```python
from build123d import *

# Parameters (mm, degrees)
SKETCH1_W             = 105.41
SKETCH1_H             = 114.3
BOSS_EXTRUDE1_DEPTH   = 3.175
F_8_CLEARANCE_HOLE1_D = 4.4958
MIRROR2_COPY_1_D      = 4.4958
CUT_EXTRUDE4_REACH    = 80.002
SKETCH15_W            = 41.275
SKETCH15_H            = 79.375
CUT_EXTRUDE5_REACH    = 80.002
SKETCH17_R            = 1.5875
CUT_EXTRUDE6_DEPTH    = 6.35


with BuildPart() as part:
    # Sketch1 → Boss-Extrude1 (new, symmetric)
    with BuildSketch(Plane(origin=(0, 0, 0), x_dir=(1, 0, 0), z_dir=(0, 1, 0))):
        Rectangle(SKETCH1_W, SKETCH1_H)
    extrude(amount=BOSS_EXTRUDE1_DEPTH, both=True)

    # #8 Clearance Hole1 (through all)
    with Locations(Plane(origin=(0, 3.175, 0), x_dir=(1, 0, 0), z_dir=(0, 1, 0))):
        with Locations((-46.355, 50.8)):
            f_8_clearance_hole1 = Hole(F_8_CLEARANCE_HOLE1_D / 2)

    # Mirror1: #8 Clearance Hole1 across plane
    add(f_8_clearance_hole1.mirror(Plane.XY), mode=Mode.SUBTRACT)

    # Mirror2: #8 Clearance Hole1 across plane
    add(f_8_clearance_hole1.mirror(Plane(origin=(0, 0, 0), x_dir=(0, 0, 1), z_dir=(1, 0, 0))), mode=Mode.SUBTRACT)

    # Mirror2 copy 1 (through all)
    with Locations(Plane(origin=(0, 3.175, 0), x_dir=(-1, 0, 0), z_dir=(0, 1, 0))):
        with Locations((-46.355, 50.8)):
            Hole(MIRROR2_COPY_1_D / 2)

    # Sketch15 → Cut-Extrude4 (cut, up to next)
    with BuildSketch(Plane.XZ.offset(3.175), mode=Mode.PRIVATE) as cut_extrude4_sk1:
        with Locations((6.6675, 4.7625)):
            Rectangle(SKETCH15_W, SKETCH15_H)
    cut_extrude4_tool1 = extrude(cut_extrude4_sk1.sketch, amount=-CUT_EXTRUDE4_REACH, mode=Mode.PRIVATE) & part.part
    add(cut_extrude4_tool1.solids().sort_by_distance((6.6675, -3.175, 4.7625))[0], mode=Mode.SUBTRACT)

    # Sketch16 → Cut-Extrude5 (cut, up to next)
    with BuildSketch(Plane(origin=(0, 3.175, 0), x_dir=(1, 0, 0), z_dir=(0, 1, 0)), mode=Mode.PRIVATE) as cut_extrude5_sk1:
        Polygon((-52.705, -6.35), (-52.705, 6.35), (-46.355, 6.35), (-46.355, 1.89865), (-42.8545625, 1.89865), (-42.8545625, 3.96875), (-40.0764375, 3.96875), (-40.0764375, 1.89865), (-36.576, 1.89865), (-36.576, -1.89865), (-40.0764375, -1.89865), (-40.0764375, -3.96875), (-42.8545625, -3.96875), (-42.8545625, -1.89865), (-46.355, -1.89865), (-46.355, -6.35), align=None)
    cut_extrude5_tool1 = extrude(cut_extrude5_sk1.sketch, amount=-CUT_EXTRUDE5_REACH, mode=Mode.PRIVATE) & part.part
    add(cut_extrude5_tool1.solids().sort_by_distance((-46.496113, 3.175, 0))[0], mode=Mode.SUBTRACT)

    # Sketch17 → Cut-Extrude6 (cut)
    with BuildSketch(Plane(origin=(0, 3.175, 0), x_dir=(1, 0, 0), z_dir=(0, 1, 0))):
        with Locations(Location((-17.145, 28.575, 0), (0, 0, 270))):
            Circle(SKETCH17_R)
        with Locations(Location((-17.145, -38.1, 0), (0, 0, 270))):
            Circle(SKETCH17_R)
        with Locations(Location((30.48, -38.1, 0), (0, 0, 90))):
            Circle(SKETCH17_R)
        with Locations(Location((30.48, 28.575, 0), (0, 0, 90))):
            Circle(SKETCH17_R)
        Polygon((-20.32, 8.73125), (-13.97, 8.73125), (-13.97, 21.43125), (-20.32, 21.43125), (-20.32, 16.9799), (-23.8204375, 16.9799), (-23.8204375, 19.05), (-26.5985625, 19.05), (-26.5985625, 16.9799), (-30.099, 16.9799), (-30.099, 13.1826), (-26.5985625, 13.1826), (-26.5985625, 11.1125), (-23.8204375, 11.1125), (-23.8204375, 13.1826), (-20.32, 13.1826), align=None)
        Polygon((33.655, -18.25625), (27.305, -18.25625), (27.305, -30.95625), (33.655, -30.95625), (33.655, -26.5049), (37.1554375, -26.5049), (37.1554375, -28.575), (39.9335625, -28.575), (39.9335625, -26.5049), (43.434, -26.5049), (43.434, -22.7076), (39.9335625, -22.7076), (39.9335625, -20.6375), (37.1554375, -20.6375), (37.1554375, -22.7076), (33.655, -22.7076), align=None)
        Polygon((-20.32, -26.5049), (-20.32, -30.95625), (-13.97, -30.95625), (-13.97, -18.25625), (-20.32, -18.25625), (-20.32, -22.7076), (-23.8204375, -22.7076), (-23.8204375, -20.6375), (-26.5985625, -20.6375), (-26.5985625, -22.7076), (-30.099, -22.7076), (-30.099, -26.5049), (-26.5985625, -26.5049), (-26.5985625, -28.575), (-23.8204375, -28.575), (-23.8204375, -26.5049), align=None)
        Polygon((33.655, 16.9799), (33.655, 21.43125), (27.305, 21.43125), (27.305, 8.73125), (33.655, 8.73125), (33.655, 13.1826), (37.1554375, 13.1826), (37.1554375, 11.1125), (39.9335625, 11.1125), (39.9335625, 13.1826), (43.434, 13.1826), (43.434, 16.9799), (39.9335625, 16.9799), (39.9335625, 19.05), (37.1554375, 19.05), (37.1554375, 16.9799), align=None)
    extrude(amount=-CUT_EXTRUDE6_DEPTH, mode=Mode.SUBTRACT)


solid = part.part
```
Verification items for the finished model (mm, model axes). A direction names the side the tool comes from. Give positions to 0.01 mm unless a question says otherwise; leave off trailing zeros. Order: outer loops, then holes, each group sorted by start corner. A loop starts at its lowest first (then second) coordinate and runs counter-clockwise, first axis right, second up. Notation, with made-up numbers: M 68,88 L 83,88 A12 cw 83,103 Z; hole C -29,44 d8. An arc over 180 degrees is marked long. Answer in a Markdown table with one row per item. Add a question column.
Item 1: Tool access check on faces 4 (the flat face through (-17, 0, -21.431)), 5 (the flat face through (-52.705, 0, -31)), 6 (the flat face through (-45, 0, -1.899)). Record the directions out of +Z, -Z, +X, -X, +Y, -Y that give a thin tool (end or side, any length) a straight path to the whole face; none if there is none.
Item 2: Section check A-A, the plane z = 38.1. Enter the section's corners in (x, y) (1 decimal).
Item 3: Mould release check, pull along Z, two halves, no side actions. Record for faces 1 (the flat face through (-38, 0, 1.899)), 2 (the flat face through (-24, -3.175, -1)), 3 (the cylindrical face through (-18.55, 0.04, -27.84)): released by +Z, released by -Z, zero draft, split by the parting line, or undercut.
Item 4: Section check B-B, the plane z = 50.8. Enter the section's corners in (x, y) (3 decimals), and give its area (3 significant figures).
Item 5: Gauge pin test, flat end, axial feed: pin 1 (3 mm diameter, centred on x = 30.48, z = -28.575, fed in from -Y). Record the tip position at first contact, or that the pin passes through.
Item 6: Section check C-C, the plane y = -0.25. State how many separate pieces and enclosed holes the cut face has, and give its area (3 significant figures).
Item 7: Scan lines: probe 1 along X at (y, z) = (0.75, 38.1) (1 decimal); probe 2 along Z at (x, y) = (-43.5, 0); probe 3 along Z at (x, y) = (24.5, 0.5) (3 decimals). Record each from-to range of solid material in increasing order. Write a range as from..to.
Filled sheet:
| question | item | result |
|---|---|---|
| 1 | face 4 | +Y, -Y |
| 1 | face 5 | +Z, -Z, -X, +Y, -Y |
| 1 | face 6 | -X, +Y, -Y |
| 2 | outline | M -52.7,-3.2 L -18.7,-3.2 L -18.7,3.2 L -52.7,3.2 Z; M -15.6,-3.2 L -14,-3.2 L -14,3.2 L -15.6,3.2 Z; M 27.3,-3.2 L 28.9,-3.2 L 28.9,3.2 L 27.3,3.2 Z; M 32.1,-3.2 L 52.7,-3.2 L 52.7,3.2 L 32.1,3.2 Z |
| 3 | face 1 | undercut |
| 3 | face 2 | zero draft |
| 3 | face 3 | undercut |
| 4 | outline | M -52.705,-3.175 L -48.603,-3.175 L -48.603,3.175 L -52.705,3.175 Z; M -44.107,-3.175 L 44.107,-3.175 L 44.107,3.175 L -44.107,3.175 Z; M 48.603,-3.175 L 52.705,-3.175 L 52.705,3.175 L 48.603,3.175 Z |
| 4 | area | 612 mm^2 |
| 5 | pin 1 | passes through |
| 6 | separate pieces | 1 |
| 6 | enclosed holes | 9 |
| 6 | area | 8,030 mm^2 |
| 7 | probe 1 | x = -52.7..-18.7, -15.6..-14, 27.3..28.9, 32.1..52.7 |
| 7 | probe 2 | z = -57.15..-1.9, 1.9..57.15 |
| 7 | probe 3 | z = -57.15..-34.925, 44.45..57.15 |
